Design review of the part shown in the three views and the two pictorial views. Dimensions are in mm from the part's minimum x, y and z. A direction names the side the tool comes from. Round coordinates to 2 decimals unless told otherwise and drop trailing zeros. Order: outer loops, then holes, each group sorted by start corner. A loop starts at its lowest first (then second) coordinate and runs counter-clockwise, first axis right, second up. Notation, with made-up numbers: (12, -29) - (28, -29) arc R18 cw to (28, 4) - close; hole circle Ø7 at (63.25, 77.25). An arc over 180 degrees is marked (long way). One line per question, with ' | ' between items. Start each with the question number.
Item 1: Add section A-A on z = 61. State the section outline as (x, y) points (3 decimals), and give its area (3 significant figures).
Item 2: Draft analysis for pull direction X (two halves, no side actions). For the marked faces 3 and 4, state which applies: +X half, -X half, draft (parallel to the pull), parting line (faces both ways), or undercut.
Item 3: Add section B-B on x = 22. State the section outline as (y, z) points.
Item 4: Add section D-D on x = 92.5. State the section outline as (y, z) points.
Item 5: For L1, parallel to X at y = 6.8, z = 72; L2, parallel to Z at x = 95, y = 6.45; L3, parallel to X at y = 2.25, z = 11.5 (3 decimals), list the stretches that pass through material, from the lowest coordinate up. Write a range as [from, to].
Item 6: Tool access review of the marked faces 1 and 2: name each direction out of +Z, -Z, +X, -X, +Y, -Y from which nothing blocks a thin tool from reaching the whole face with its end or side.
Item 7: Insertion check: pin 1 Ø1.2 at (x, z) = (5, 12) entering from -Y; pin 2 Ø10 at (x, z) = (70, 12.5) entering from +Y; pin 3 Ø1.2 at (y, z) = (2.5, 17) entering from +X (3 decimals). Each pin has a flat end and moves straight along its axis. Give the tip position at first contact, or say it passes through.
Item 8: Add section C-C on z = 39. State the section outline as (x, y) points.
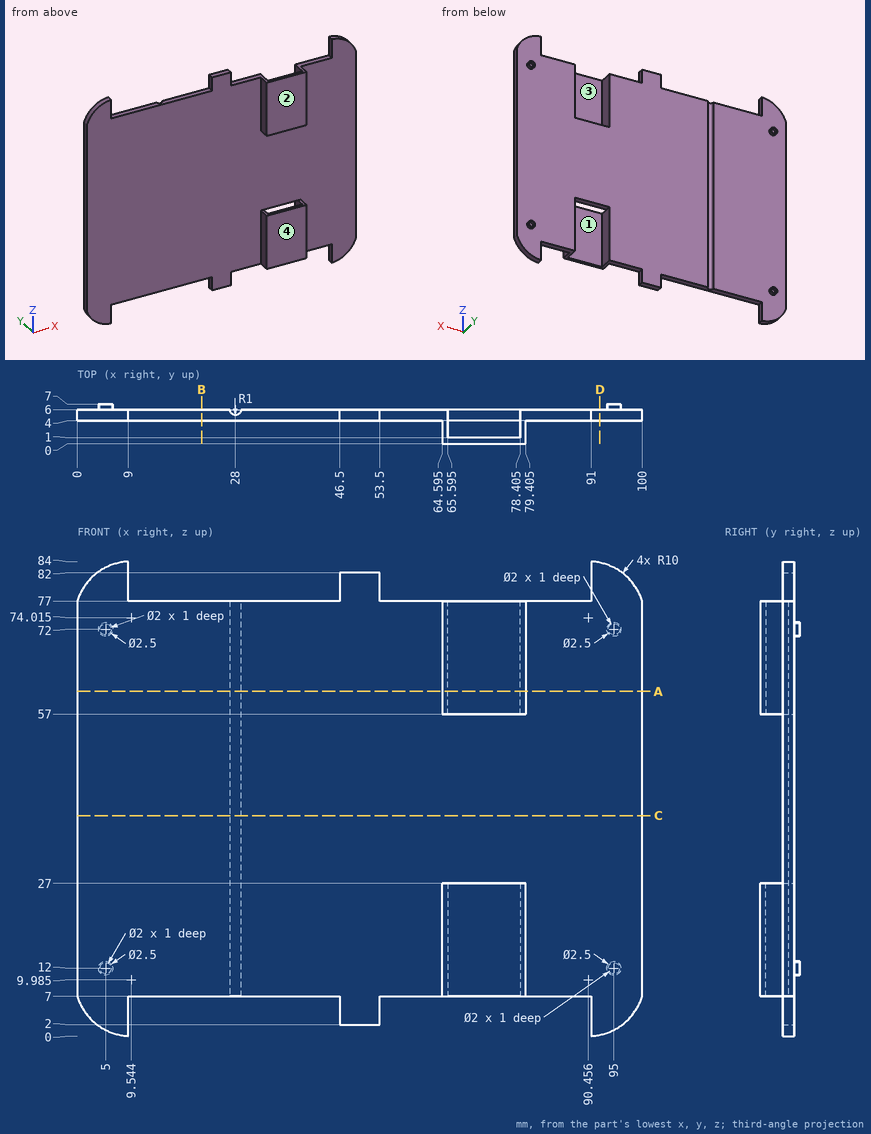
Determined:
1) outline: (0, 4) - (64.595, 4) - (64.595, 0) - (79.405, 0) - (79.405, 4) - (100, 4) - (100, 6) - (78.405, 6) - (78.405, 1) - (65.595, 1) - (65.595, 6) - (29, 6) arc R1 cw to (27, 6) - (0, 6) - close | area: 194 mm2
2) face 3: undercut | face 4: draft
3) outline: (4, 7) - (6, 7) - (6, 77) - (4, 77) - close
4) outline: (4, 0.2) - (6, 0.2) - (6, 83.8) - (4, 83.8) - close
5) L1: [3.75, 4], [6, 6.25], [93.75, 94], [96, 96.25] | L2: [10.75, 11], [13, 13.25], [70.75, 71], [73, 73.25] | L3: [64.595, 65.595], [78.405, 79.405]
6) face 1: +Z, -Z, +Y | face 2: +Z, -Z, +X, -X, -Y
7) pin 1: y = 4 | pin 2: y = 6 | pin 3: x = 79.405
8) outline: (0, 4) - (100, 4) - (100, 6) - (29, 6) arc R1 cw to (27, 6) - (0, 6) - close
